Input: dimensioned drawing with shaded views. Units: mm. Origin: part minimum x, y, z. A direction names the side the tool comes from. Round coordinates to 2 decimals unless told otherwise and drop trailing zeros. Order: outer loops, then holes, each group sorted by start corner. A loop starts at its lowest first (then second) coordinate and runs counter-clockwise, first axis right, second up. Notation, with made-up numbers: (-19.5, 83) - (-6.5, 83) arc R17 cw to (-6.5, 100) - close; hole circle Ø11 at (46, -10). An arc over 180 degrees is marked (long way). Return JSON: item names as keys, results as strings. Group by question number.
1) Contact query for a flat-ended pin moving along its axis: P1, Ø5, axis at x = 40.5, z = 2, coming from the -Y side. Output: stop coordinate, or through.
2) Section B-B, the plane x = 26.5. Return loops of the section in (y, z).
3) Mould query, pull axis Y, two halves, no side actions, for the marked faces 1, 2 and 3. Classes: pulls with the +Y half, pulls with the -Y half, needs draft (parallel to the pull), parting line crosses it, or undercut.
4) Section D-D, the plane z = 15. Return loops of the section in (x, y), plus the area to 3 significant figures.
5) Ray query, line 1 (X direction, y = 14.75, z = 15.25); line 2 (Z direction, x = 22, y = 25.5); line 3 (Z direction, x = 49, y = 24.5). Return the intervals inside material, ascending. Write a range as from..to.
6) Section C-C, the plane y = 14. Give the number of separate pieces and of enclosed holes in the cut face, plus the area to 3 significant figures.
7) Access query for the marked faces 4, 5 and 6. Directions: +Z, -Z, +X, -X, +Y, -Y. A direction counts if a zero-diameter tool reaches every point of the face in a straight line with its end or side. Return the directions, or none.
8) Section A-A, the plane y = 26. Return loops of the section in (x, z), plus the area to 3 significant figures.
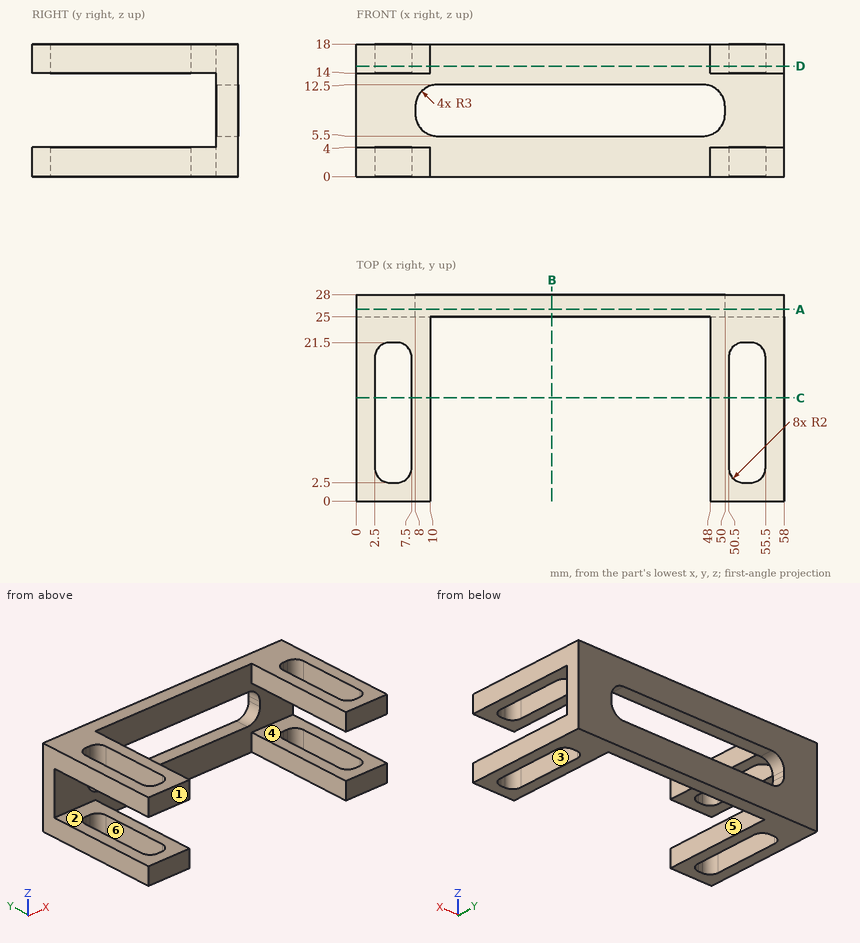
Geometry check:
{
 "1": {"P1": "y = 25"},
 "2": {"outline": "(25, 0) - (28, 0) - (28, 5.5) - (25, 5.5) - close; (25, 12.5) - (28, 12.5) - (28, 18) - (25, 18) - close"},
 "3": {"face 1": "pulls with the -Y half", "face 2": "needs draft", "face 3": "undercut"},
 "4": {"outline": "(0, 0) - (10, 0) - (10, 25) - (48, 25) - (48, 0) - (58, 0) - (58, 28) - (0, 28) - close; hole (2.5, 4.5) arc R2 ccw to (4.5, 2.5) - (5.5, 2.5) arc R2 ccw to (7.5, 4.5) - (7.5, 19.5) arc R2 ccw to (5.5, 21.5) - (4.5, 21.5) arc R2 ccw to (2.5, 19.5) - close; hole (50.5, 4.5) arc R2 ccw to (52.5, 2.5) - (53.5, 2.5) arc R2 ccw to (55.5, 4.5) - (55.5, 19.5) arc R2 ccw to (53.5, 21.5) - (52.5, 21.5) arc R2 ccw to (50.5, 19.5) - close", "area": "491 mm2"},
 "5": {"line 1": "0..2.5, 7.5..10, 48..50.5, 55.5..58", "line 2": "0..5.5, 12.5..18", "line 3": "0..4, 14..18"},
 "6": {"separate pieces": "8", "enclosed holes": "0", "area": "80.0 mm2"},
 "7": {"face 4": "+X, -X, -Y", "face 5": "+Z, -Z, -Y", "face 6": "+Z, -Z"},
 "8": {"outline": "(0, 0) - (58, 0) - (58, 18) - (0, 18) - close; hole (8, 8.5) arc R3 ccw to (11, 5.5) - (47, 5.5) arc R3 ccw to (50, 8.5) - (50, 9.5) arc R3 ccw to (47, 12.5) - (11, 12.5) arc R3 ccw to (8, 9.5) - close", "area": "758 mm2"}
}
